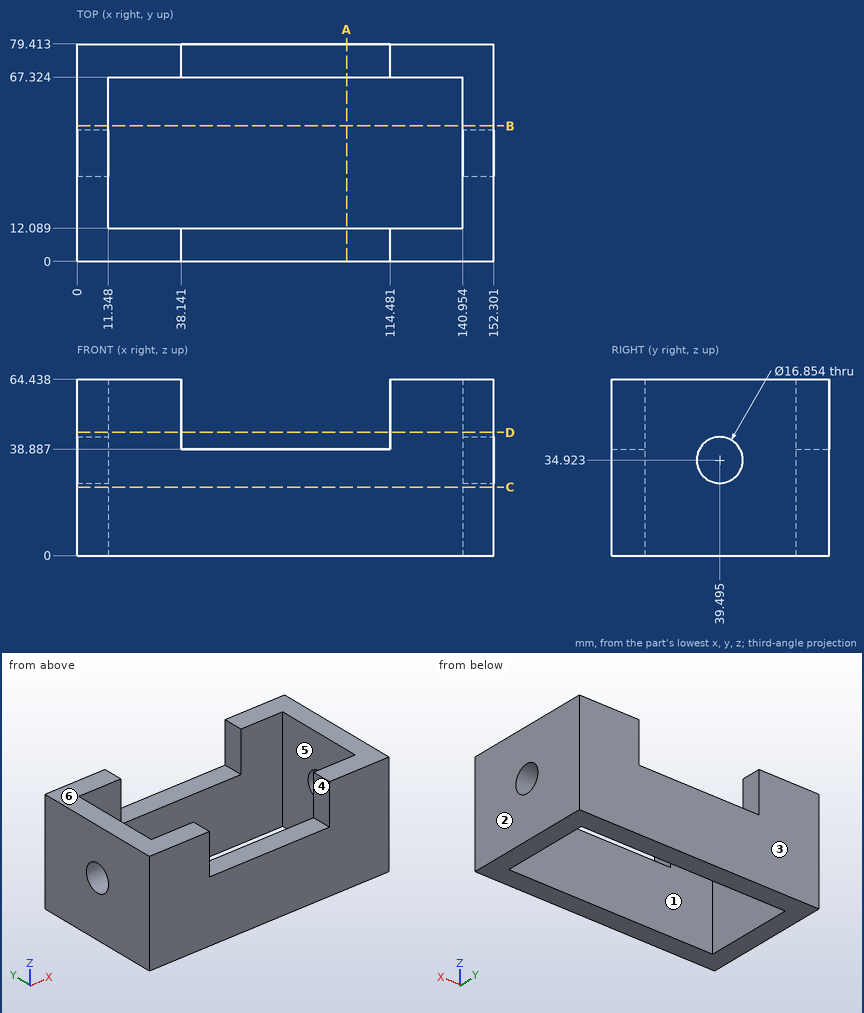
Verification items for this drawing (mm, ordinates from the low corner). A direction names the side the tool comes from. Round coordinates to 2 decimals unless told otherwise and drop trailing zeros. Order: outer loops, then holes, each group sorted by start corner. A loop starts at its lowest first (then second) coordinate and runs counter-clockwise, first axis right, second up. Notation, with made-up numbers: M -12.75,-28 L 10.25,-28 A32 ccw 10.25,8 Z; hole C 88,88 d10. An arc over 180 degrees is marked long. Answer in a Markdown table with one row per item. Add a question column.
Item 1: Set-up check for the marked faces 4, 5 and 6: record each of +Z, -Z, +X, -X, +Y, -Y from which the full face is reachable in a straight line by a thin tool's end or side.
Item 2: Material ranges on L1, parallel to Y at x = 119, z = 31.5; L2, parallel to X at y = 55, z = 18; L3, parallel to X at y = 6.5, z = 51.5, recorded low to high. Write a range as [from, to].
Item 3: Draft check along Y on the marked faces 1, 2 and 3. Enter one of: released by +Y, released by -Y, zero draft, split by the parting line, or undercut.
Item 4: Depth check by flat-ended pin: pin 1 Ø9.5 at (x, y) = (66, 4) entering from +Z. Enter the tip coordinate at first touch or a pass-through.
Item 5: Sectioned sample at B-B, the plane y = 49.5. Enter the section's corners in (x, z), plus the area to 3 significant figures.
Item 6: Sectioned sample at C-C, the plane z = 25. Enter the section's corners in (x, y), plus the area to 3 significant figures.
Item 7: Sectioned sample at D-D, the plane z = 45. Enter the section's corners in (x, y).
Item 8: Sectioned sample at A-A, the plane x = 98.5. Enter the section's corners in (y, z).
Filled in:
| question | item | result |
|---|---|---|
| 1 | face 4 | +Z, +Y, -Y |
| 1 | face 5 | +Z, -Z |
| 1 | face 6 | +Z, +X, -X, +Y, -Y |
| 2 | L1 | y = [0, 12.09], [67.32, 79.41] |
| 2 | L2 | x = [0, 11.35], [140.95, 152.3] |
| 2 | L3 | x = [0, 38.14], [114.48, 152.3] |
| 3 | face 1 | undercut |
| 3 | face 2 | zero draft |
| 3 | face 3 | released by +Y |
| 4 | pin 1 | stops at z = 38.89 |
| 5 | outline | M 0,0 L 11.35,0 L 11.35,64.44 L 0,64.44 Z; M 140.95,0 L 152.3,0 L 152.3,64.44 L 140.95,64.44 Z |
| 5 | area | 1,460 mm² |
| 6 | outline | M 0,0 L 152.3,0 L 152.3,79.41 L 0,79.41 Z; hole M 11.35,12.09 L 140.95,12.09 L 140.95,67.32 L 11.35,67.32 Z |
| 6 | area | 4,940 mm² |
| 7 | outline | M 0,0 L 38.14,0 L 38.14,12.09 L 11.35,12.09 L 11.35,67.32 L 38.14,67.32 L 38.14,79.41 L 0,79.41 Z; M 114.48,0 L 152.3,0 L 152.3,79.41 L 114.48,79.41 L 114.48,67.32 L 140.95,67.32 L 140.95,12.09 L 114.48,12.09 Z |
| 8 | outline | M 0,0 L 12.09,0 L 12.09,38.89 L 0,38.89 Z; M 67.32,0 L 79.41,0 L 79.41,38.89 L 67.32,38.89 Z |
